from build123d import *

# Parameters (mm, degrees)
SKETCH1_R           = 3
BOSS_EXTRUDE1_DEPTH = 2.5
SKETCH2_R           = 1.5
BOSS_EXTRUDE2_DEPTH = 5.5
CHAMFER1_SIZE       = 2.5
CUT_EXTRUDE1_DEPTH  = 1


with BuildPart() as part:
    # Sketch1 → Boss-Extrude1 (new body)
    with BuildSketch(Plane(origin=(0, 0, 0), x_dir=(1, 0, 0), z_dir=(0, 1, 0))):
        with Locations(Location((0, 0, 0), (0, 0, 270))):
            Circle(SKETCH1_R)
    extrude(amount=BOSS_EXTRUDE1_DEPTH)

    # Sketch2 → Boss-Extrude2 (add)
    with BuildSketch(Plane(origin=(0, 2.5, 0), x_dir=(1, 0, 0), z_dir=(0, 1, 0))):
        with Locations(Location((0, 0, 0), (0, 0, 270))):
            Circle(SKETCH2_R)
    extrude(amount=BOSS_EXTRUDE2_DEPTH)

    # Chamfer1
    # the kernel refuses this chamfer: 2.5 mm, written as the material it takes off along each edge
    with BuildSketch(Plane(origin=(0, 2.5, 0), x_dir=(0, 0, 1), z_dir=(-1, 0, 0))) as chamfer1_piece_1_section:
        Polygon((3, -CHAMFER1_SIZE), (3 - CHAMFER1_SIZE, 0), (3, 0), align=None)
    chamfer1_piece_1 = revolve(axis=Axis((0, 2.5, 0), (0, 1, 0)), mode=Mode.PRIVATE)
    chamfer1_piece_1 = chamfer1_piece_1 - Plane(origin=(0, 0.739386172, 0), x_dir=(0, 0, 1), z_dir=(0, -1, 0)) * Cylinder(1.5, 12, mode=Mode.PRIVATE)
    add(chamfer1_piece_1, mode=Mode.SUBTRACT)

    # Sketch3 → Cut-Extrude1 (cut)
    with BuildSketch(Plane.XZ):
        Polygon((1.251191911, -0.896964433), (1.402389941, 0.635081763), (0.15119803, 1.532046196), (-1.251191911, 0.896964433), (-1.402389941, -0.635081763), (-0.15119803, -1.532046196), align=None)
    extrude(amount=-CUT_EXTRUDE1_DEPTH, mode=Mode.SUBTRACT)


solid = part.part
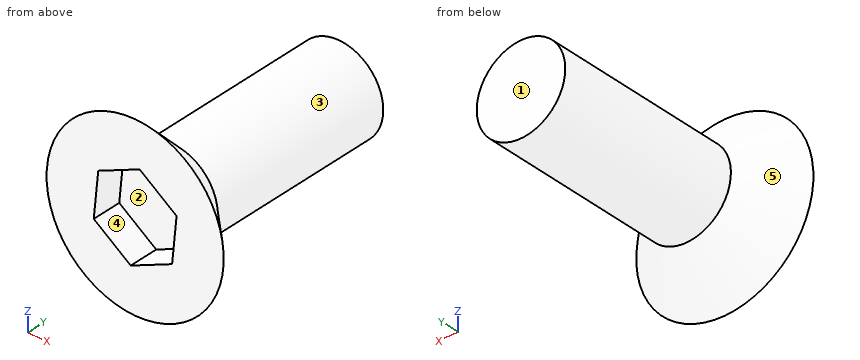
CAD build for the part. Positions are in the model's coordinates, mm. Face numbers are marked on the shaded views. A direction names the side the tool comes from. Give positions to 0.01 mm unless a question says otherwise; leave off trailing zeros. Write each loop counter-clockwise with the first axis right and the second up, starting at its lowest first coordinate (ties: lowest second). Pieces come first, ordered by that corner, then holes. Notation, with made-up numbers: M 42.5,56.25 L 69.5,56.25 A23 ccw 69.5,83.25 Z; hole C -37.75,-15 d8. An arc over 180 degrees is marked long. Put each result on its own line as item: value. Start each with the question number.
(1) Band-saw the part on B-B, the plane y = 4. Write the cut outline in (x, z), and give its area (3 significant figures).
(2) Band-saw the part on C-C, the plane z = 0. Write the cut outline in (x, y), and give its area (3 significant figures).
(3) Probe L1, parallel to X at y = 6.75, z = -1.2; L2, parallel to Y at x = -0.3, z = -0.55; L3, parallel to X at y = 2.25, z = 0.15. List the from-to ranges inside material, lowest first.
(4) Which spindle directions (+Z, -Z, +X, -X, +Y, -Y) get a long thin tool onto all of the face, cutting with end or side? Do the marked faces 4 and 5. Say none if no direction does.
(5) Band-saw the part on A-A, the plane x = 0. Write the cut outline in (y, z).
(6) Flat gauge pins, fed straight in: pin 1 Ø2 at (x, z) = (-1.5, 1) entering from -Y; pin 2 Ø1.5 at (y, z) = (6.5, 2) entering from +X; pin 3 Ø1.4 at (x, z) = (0, 0) entering from -Y; pin 4 Ø1 at (x, y) = (-1.5, 2) entering from +Z. Where does each tip first touch, or does it go through?
(7) Mould opens along X. For the marked faces 1, 2 and 3 say: +X half, -X half, draft (parallel to the pull), parting line (faces both ways), or undercut.
Response values:
1. outline: C 0,0 d3
1. area: 7.07 mm2
2. outline: M -3,0 L -1.34,0 L -1.34,1 L 1.34,1 L 1.34,0 L 3,0 L 1.5,1.5 L 1.5,8 L -1.5,8 L -1.5,1.5 Z
2. area: 23.6 mm2
3. L1: x = -0.9 to 0.9
3. L2: y = 1 to 8
3. L3: x = -1.49 to 1.49
4. face 4: -Y
4. face 5: +Y
5. outline: M 0,-3 L 1.5,-1.5 L 8,-1.5 L 8,1.5 L 1.5,1.5 L 0,3 L 0,1.46 L 1,1.46 L 1,-1.46 L 0,-1.46 Z
6. pin 1: stops at y = 0
6. pin 2: stops at x = 0.83
6. pin 3: stops at y = 1
6. pin 4: stops at z = 1.12
7. face 1: draft
7. face 2: undercut
7. face 3: parting line
